from build123d import *

# Parameters (mm, degrees)
BASE_W            = 45
BASE_H            = 45
BLOCK_DEPTH       = 15
SKETCH5_W         = 1.2
SKETCH5_H         = 15
ROW_1_SEED_DEPTH  = 66.383484153
ROW_1_START       = 25
ROW_1_OUTLINE_W   = 2.1
ROW_1_OUTLINE_H   = 15
ROW_1_OUTLINE_W_2 = 1.8
ROW_1_OUTLINE_W_3 = 1.5
ROW_1_DEPTH       = 15
SKETCH6_W         = 2.4
SKETCH6_H         = 15
ROW_2_SEED_DEPTH  = 66.383484153
ROW_2_START       = 5
ROW_2_OUTLINE_W   = 3
ROW_2_OUTLINE_H   = 15
ROW_2_OUTLINE_W_2 = 2.7
ROW_2_DEPTH       = 15
SKETCH8_W         = 45
SKETCH8_H         = 3
ADAPTER_DEPTH     = 10


# Read off the part's stored shape, not the designer's step: row-1, row-2
with BuildPart() as part:
    # base → block (new body)
    with BuildSketch(Plane.XY):
        with Locations((22.5, 22.5)):
            Rectangle(BASE_W, BASE_H)
    extrude(amount=BLOCK_DEPTH)

    # Sketch5 → row-1-seed (cut, through all)
    with BuildSketch(Plane.XY.offset(15)):
        with Locations((5.6, 32.5)):
            Rectangle(SKETCH5_W, SKETCH5_H)
        with Locations((8, 32.5)):
            Rectangle(SKETCH5_W, SKETCH5_H)
    extrude(amount=-ROW_1_SEED_DEPTH, mode=Mode.SUBTRACT)

    # row-1 outline → row-1 (cut)
    with BuildSketch(Plane(origin=(0, 0, 0), x_dir=(1, 0, 0), z_dir=(0, 1, 0)).offset(ROW_1_START)):
        with Locations((38.75, -7.5)):
            Rectangle(ROW_1_OUTLINE_W, ROW_1_OUTLINE_H)
        with Locations((34.55, -7.5)):
            Rectangle(ROW_1_OUTLINE_W, ROW_1_OUTLINE_H)
        with Locations((27.6, -7.5)):
            Rectangle(ROW_1_OUTLINE_W_2, ROW_1_OUTLINE_H)
        with Locations((24, -7.5)):
            Rectangle(ROW_1_OUTLINE_W_2, ROW_1_OUTLINE_H)
        with Locations((17.35, -7.5)):
            Rectangle(ROW_1_OUTLINE_W_3, ROW_1_OUTLINE_H)
        with Locations((14.35, -7.5)):
            Rectangle(ROW_1_OUTLINE_W_3, ROW_1_OUTLINE_H)
    extrude(amount=ROW_1_DEPTH, mode=Mode.SUBTRACT)

    # Sketch6 → row-2-seed (cut, through all)
    with BuildSketch(Plane.XY.offset(15)):
        with Locations((6.2, 12.5)):
            Rectangle(SKETCH6_W, SKETCH6_H)
        with Locations((11, 12.5)):
            Rectangle(SKETCH6_W, SKETCH6_H)
    extrude(amount=-ROW_2_SEED_DEPTH, mode=Mode.SUBTRACT)

    # row-2 outline → row-2 (cut)
    with BuildSketch(Plane(origin=(0, 0, 0), x_dir=(1, 0, 0), z_dir=(0, 1, 0)).offset(ROW_2_START)):
        with Locations((37.8, -7.5)):
            Rectangle(ROW_2_OUTLINE_W, ROW_2_OUTLINE_H)
        with Locations((31.8, -7.5)):
            Rectangle(ROW_2_OUTLINE_W, ROW_2_OUTLINE_H)
        with Locations((23.95, -7.5)):
            Rectangle(ROW_2_OUTLINE_W_2, ROW_2_OUTLINE_H)
        with Locations((18.55, -7.5)):
            Rectangle(ROW_2_OUTLINE_W_2, ROW_2_OUTLINE_H)
    extrude(amount=ROW_2_DEPTH, mode=Mode.SUBTRACT)

    # Sketch8 → adapter (add)
    with BuildSketch(Plane(origin=(0, 0, 0), x_dir=(-1, 0, 0), z_dir=(0, 0, -1))):
        with Locations((-22.5, 31.5)):
            Rectangle(SKETCH8_W, SKETCH8_H)
        with Locations((-22.5, 13.5)):
            Rectangle(SKETCH8_W, SKETCH8_H)
    extrude(amount=ADAPTER_DEPTH)


solid = part.part
Build history of the part. All positions in model axes, mm. A direction names the side the tool comes from. Give positions to 0.01 mm unless a question says otherwise; leave off trailing zeros. Order: outer loops, then holes, each group sorted by start corner. A loop starts at its lowest first (then second) coordinate and runs counter-clockwise, first axis right, second up. Notation, with made-up numbers: M -18,69 L -14,69 A14 ccw -14,77 Z; hole C 45.5,47.5 d10. An arc over 180 degrees is marked long. Use one line per item in the form item = value.
1) Saw through at B-B (y = 16). Give the cut face in (x, z).
Calculated:
outline = M 0,0 L 5,0 L 5,15 L 0,15 Z; M 7.4,0 L 9.8,0 L 9.8,15 L 7.4,15 Z; M 12.2,0 L 17.2,0 L 17.2,15 L 12.2,15 Z; M 19.9,0 L 22.6,0 L 22.6,15 L 19.9,15 Z; M 25.3,0 L 30.3,0 L 30.3,15 L 25.3,15 Z; M 33.3,0 L 36.3,0 L 36.3,15 L 33.3,15 Z; M 39.3,0 L 45,0 L 45,15 L 39.3,15 Z
2) Drop flat-ended pins along their axis: pin 1 (2 mm diameter, centred on x = 23.5, y = 14, fed in from +Z); pin 2 (5 mm diameter, centred on x = 7, z = -4, fed in from +Y). Give the stop position or say it passes through.
Calculated:
pin_1 = 15
pin_2 = 33
3) Tool access for faces 4 (the face through (23.1, 32, 8)), 5 (the face through (32, 20, 7)), 6 (the face through (23, 15, -5)): list every direction of +Z, -Z, +X, -X, +Y, -Y with a clear straight run to the whole face (end or side of a thin tool).
Calculated:
face_4 = +Z
face_5 = +Z, -Z
face_6 = -Z, +X, -X
4) Saw through at C-C (x = 8). Give the cut face in (y, z).
Calculated:
outline = M 0,0 L 12,0 L 12,-10 L 15,-10 L 15,0 L 25,0 L 25,15 L 0,15 Z; M 30,-10 L 33,-10 L 33,0 L 30,0 Z; M 40,0 L 45,0 L 45,15 L 40,15 Z
5) Two-plate mould, pull along Y, no slides. Class faces 1 (the face through (22, 45, 7)), 2 (the face through (22, 23, 15)), 3 (the face through (19, 5, 7)): released by +Y, released by -Y, zero draft, split by the parting line, or undercut.
Calculated:
face_1 = released by +Y
face_2 = zero draft
face_3 = undercut
6) Saw through at A-A (z = -4). Give the cut face in (x, y), plus the area to 3 significant figures.
Calculated:
outline = M 0,12 L 45,12 L 45,15 L 0,15 Z; M 0,30 L 45,30 L 45,33 L 0,33 Z
area = 270 mm2
7) Saw through at D-D (x = 40.5). Give the cut face in (y, z).
Calculated:
outline = M 0,0 L 12,0 L 12,-10 L 15,-10 L 15,0 L 30,0 L 30,-10 L 33,-10 L 33,0 L 45,0 L 45,15 L 0,15 Z
8) Probe probe 1 along Y at (x, z) = (14, -7.5); probe 2 along Y at (x, z) = (14, 0.25); probe 3 along Z at (x, y) = (11, 38). List the from-to ranges inside material, lowest first.
Calculated:
probe_1 = 12 to 15, 30 to 33
probe_2 = 0 to 25, 40 to 45
probe_3 = 0 to 15
